Part model, mm, in its own coordinate system. A direction names the side the tool comes from. Give positions to 0.01 mm unless a question says otherwise; leave off trailing zeros. Write each loop counter-clockwise with the first axis right and the second up, starting at its lowest first coordinate (ties: lowest second). Pieces come first, ordered by that corner, then holes. Notation, with made-up numbers: M 61.25,-4 L 73.25,-4 A19 ccw 73.25,24 Z; hole C -14.5,-24 d10. An arc over 180 degrees is marked long. Use CSV: the item, a comma, the result in double quotes. Start each with the question number.
1. Drill centre lines: line 1 along X through (y, z) = (12.7, -8.2); line 2 along Y through (x, z) = (1.5, -3); line 3 along X through (y, z) = (5, -3.25). Where is each one in solid material? Low to high. Write a range as from..to.
2. Band-saw the part on C-C, the plane z = -3.75. List the corners of the cut face in (x, y).
3. 3-axis set-ups, long thin cutter, end or side, ignore diameter. For faces 4 (the face through (0, 7, -7)), 5 (the face through (6, 11, -6.604)): which of +Z, -Z, +X, -X, +Y, -Y reach the whole face in a straight line?
4. Band-saw the part on B-B, the plane x = 8.25. List the corners of the cut face in (y, z), then the cut area to 3 significant figures.
5. Band-saw the part on A-A, the plane y = 12.7. List the corners of the cut face in (x, z), then the cut area to 3 significant figures.
6. Drop a flat-ended pin along its axis: pin 1 Ø2 at (x, z) = (6, -2.5) entering from +Y. Give the stop position or say it passes through.
7. Mould opens along Z. For faces 1 (the face through (4.8, 3.2, -2.6)), 2 (the face through (6, 17.78, -8)), 3 (the face through (6, 3, 0)) say: pulls with the +Z half, pulls with the -Z half, needs draft (parallel to the pull), parting line crosses it, or undercut.
8. Band-saw the part on D-D, the plane y = 6. List the corners of the cut face in (x, z).
from build123d import *

# Parameters (mm, degrees)
SKETCH1_W           = 12.192
SKETCH1_H           = 9.779
BOSS_EXTRUDE1_DEPTH = 6.35
SKETCH2_W           = 12.192
SKETCH2_H           = 3.175
BOSS_EXTRUDE2_DEPTH = 11.43
SKETCH3_R           = 1.4732
CUT_EXTRUDE2_DEPTH  = 6.35
SKETCH4_R           = 1.4732
CUT_EXTRUDE3_DEPTH  = 6.35
SKETCH5_R           = 1.4732
CUT_EXTRUDE4_DEPTH  = 6.35


with BuildPart() as part:
    # Sketch1 → Boss-Extrude1 (new body)
    with BuildSketch(Plane(origin=(0, 0, 0), x_dir=(1, 0, 0), z_dir=(0, 1, 0))):
        with Locations((6.096, 4.8895)):
            Rectangle(SKETCH1_W, SKETCH1_H)
    extrude(amount=BOSS_EXTRUDE1_DEPTH)

    # Sketch2 → Boss-Extrude2 (add)
    with BuildSketch(Plane(origin=(0, 6.35, 0), x_dir=(1, 0, 0), z_dir=(0, 1, 0))):
        with Locations((6.096, 8.1915)):
            Rectangle(SKETCH2_W, SKETCH2_H)
    extrude(amount=BOSS_EXTRUDE2_DEPTH)

    # Sketch3 → Cut-Extrude2 (cut)
    with BuildSketch(Plane(origin=(0, 6.35, 0), x_dir=(1, 0, 0), z_dir=(0, 1, 0))):
        with Locations((25.4, 3.302)):
            Circle(SKETCH3_R)
        with Locations(Location((6.096, 3.302, 0), (0, 0, 270))):
            Circle(SKETCH3_R)
    extrude(amount=-CUT_EXTRUDE2_DEPTH, mode=Mode.SUBTRACT)

    # Sketch4 → Cut-Extrude3 (cut)
    with BuildSketch(Plane(origin=(0, 0, -9.779), x_dir=(-1, 0, 0), z_dir=(0, 0, -1))):
        with Locations((-5.207, 12.7)):
            Circle(SKETCH4_R)
    extrude(amount=-CUT_EXTRUDE3_DEPTH, mode=Mode.SUBTRACT)

    # Sketch5 → Cut-Extrude4 (cut)
    with BuildSketch(Plane(origin=(0, 0, -9.779), x_dir=(-1, 0, 0), z_dir=(0, 0, -1))):
        with Locations((-7.112, 12.7)):
            Circle(SKETCH5_R)
    extrude(amount=-CUT_EXTRUDE4_DEPTH, mode=Mode.SUBTRACT)


solid = part.part
Output:
1,line 1,"x = 0..3.73, 8.59..12.19"
1,line 2,"y = 0..6.35"
1,line 3,"x = 0..4.62, 7.57..12.19"
2,outline,"M 0,0 L 4.69,0 L 4.69,6.35 L 0,6.35 Z; M 7.5,0 L 12.19,0 L 12.19,6.35 L 7.5,6.35 Z"
3,face 4,"+Z, -Z, -X, +Y, -Y"
3,face 5,"+Z, +X, -X, +Y"
4,outline,"M 0,-9.78 L 11.76,-9.78 L 11.76,-6.6 L 6.35,-6.6 L 6.35,0 L 0,0 Z; M 13.64,-9.78 L 17.78,-9.78 L 17.78,-6.6 L 13.64,-6.6 Z"
4,area,"92.4 mm²"
5,outline,"M 0,-9.78 L 3.73,-9.78 L 3.73,-6.6 L 0,-6.6 Z; M 8.59,-9.78 L 12.19,-9.78 L 12.19,-6.6 L 8.59,-6.6 Z"
5,area,"23.3 mm²"
6,pin 1,"stops at y = 6.35"
7,face 1,"undercut"
7,face 2,"needs draft"
7,face 3,"pulls with the +Z half"
8,outline,"M 0,-9.78 L 12.19,-9.78 L 12.19,0 L 0,0 Z; hole C 6.1,-3.3 d2.95"
